from build123d import *

# Parameters (mm, degrees)
SKETCH1_W                      = 12
SKETCH1_H                      = 10.5
BASE_DEPTH                     = 8.25
CONTACT_OPENING_DEPTH          = 9
CONTACT_OPENING_LEAD_IN_SIZE   = 0.5
SKETCH3_W                      = 5.6
SKETCH3_H                      = 3.18
CONTACT_AREA_DEPTH             = 8.5
CONTACT_AREA_LEAD_IN_SIZE      = 0.5
HOLDING_TINES_DEPTH            = 1.75
CONTACT_DEPTH                  = 0.375
CONTACT_PATTERN_COUNT          = 2
CONTACT_PATTERN_PITCH          = 2.5
TH_GROUND_LEGS_DEPTH           = 0.975
TH_GROUND_LEG_SHAPE_DEPTH      = 8.43
TH_GROUND_LEG_SHAPE_DEPTH_BACK = 8.43
TH_TAILS_DEPTH                 = 0.125
TH_TAILS_PATTERN_COUNT         = 2
TH_TAILS_PATTERN_PITCH         = 2


with BuildPart() as part:
    # Sketch1 → Base (new body, symmetric)
    with BuildSketch(Plane.XY):
        Rectangle(SKETCH1_W, SKETCH1_H)
    extrude(amount=BASE_DEPTH, both=True)

    # Sketch2 → Contact Opening (cut)
    with BuildSketch(Plane.XY.offset(8.25)):
        with BuildLine():
            Line((-2.975, 4.33), (-4.225, 3.08))
            Line((-4.225, 3.08), (-4.225, -2.95))
            ThreePointArc((-4.225, -2.95), (-4.078553391, -3.303553391), (-3.725, -3.45))
            Line((-3.725, -3.45), (3.725, -3.45))
            ThreePointArc((3.725, -3.45), (4.078553391, -3.303553391), (4.225, -2.95))
            Line((4.225, -2.95), (4.225, 3.08))
            Line((4.225, 3.08), (2.975, 4.33))
            Line((2.975, 4.33), (-2.975, 4.33))
        make_face()
    extrude(amount=-CONTACT_OPENING_DEPTH, mode=Mode.SUBTRACT)

    # Contact Opening Lead-in
    contact_opening_lead_in_edges = [part.edges().sort_by_distance(p)[0] for p in [
        (0, 4.33, 8.25),
        (-3.6, 3.705, 8.25),
        (-4.225, 0.065, 8.25),
        (-4.078553391, -3.303553391, 8.25),
        (0, -3.45, 8.25),
        (4.078553391, -3.303553391, 8.25),
        (4.225, 0.065, 8.25),
        (3.6, 3.705, 8.25),
    ]]
    chamfer(contact_opening_lead_in_edges, length=CONTACT_OPENING_LEAD_IN_SIZE)

    # Sketch3 → Contact Area (add)
    with BuildSketch(Plane.XY.offset(-0.75)):
        with Locations((0, 0.44)):
            Rectangle(SKETCH3_W, SKETCH3_H)
    extrude(amount=CONTACT_AREA_DEPTH)

    # Contact Area Lead-in
    contact_area_lead_in_edges = [part.edges().sort_by_distance(p)[0] for p in [
        (-2.8, 0.44, 7.75),
        (0, -1.15, 7.75),
        (2.8, 0.44, 7.75),
        (0, 2.03, 7.75),
    ]]
    chamfer(contact_area_lead_in_edges, length=CONTACT_AREA_LEAD_IN_SIZE)

    # Sketch7 → Holding Tines (add, symmetric)
    with BuildSketch(Plane(origin=(0, 0, 0), x_dir=(1, 0, 0), z_dir=(0, 1, 0))):
        with BuildLine():
            Line((-4.225, -7.75), (-3.215243234, -5.051316752))
            ThreePointArc((-3.215243234, -5.051316752), (-3.027350135, -3.881276433), (-3.307189725, -2.729760924))
            Line((-3.307189725, -2.729760924), (-3.695, -1.9))
            Line((-3.695, -1.9), (-3.853538933, -1.974097279))
            Line((-3.853538933, -1.974097279), (-3.465728658, -2.803858203))
            ThreePointArc((-3.465728658, -2.803858203), (-3.202213044, -3.888201975), (-3.379145712, -4.989989942))
            Line((-3.379145712, -4.989989942), (-4.388902478, -7.688673189))
            Line((-4.388902478, -7.688673189), (-4.225, -7.75))
        make_face()
        with BuildLine():
            Line((4.225, -7.75), (4.388902478, -7.688673189))
            Line((4.388902478, -7.688673189), (3.379145712, -4.989989942))
            ThreePointArc((3.379145712, -4.989989942), (3.202213044, -3.888201975), (3.465728658, -2.803858203))
            Line((3.465728658, -2.803858203), (3.853538933, -1.974097279))
            Line((3.853538933, -1.974097279), (3.695, -1.9))
            Line((3.695, -1.9), (3.307189725, -2.729760924))
            ThreePointArc((3.307189725, -2.729760924), (3.027350135, -3.881276433), (3.215243234, -5.051316752))
            Line((3.215243234, -5.051316752), (4.225, -7.75))
        make_face()
    extrude(amount=HOLDING_TINES_DEPTH, both=True)

    # Sketch8 → Contact (add, symmetric)
    with BuildSketch(Plane(origin=(-1.25, 0, 0), x_dir=(0, 0, -1), z_dir=(1, 0, 0))):
        with BuildLine():
            Line((0.75, 2.03), (-2.695251124, 2.678262825))
            ThreePointArc((-2.695251124, 2.678262825), (-3.57053143, 2.712827451), (-4.418484282, 2.493086043))
            Line((-4.418484282, 2.493086043), (-5.75, 1.93))
            Line((-5.75, 1.93), (-5.681838417, 1.768819981))
            Line((-5.681838417, 1.768819981), (-4.350322699, 2.331906024))
            ThreePointArc((-4.350322699, 2.331906024), (-3.551833763, 2.538829183), (-2.727611475, 2.506280827))
            Line((-2.727611475, 2.506280827), (0.717639649, 1.858018002))
            Line((0.717639649, 1.858018002), (0.75, 2.03))
        make_face()
        with BuildLine():
            Line((-5.681838417, -0.888819981), (-5.75, -1.05))
            Line((-5.75, -1.05), (-4.418484282, -1.613086043))
            ThreePointArc((-4.418484282, -1.613086043), (-3.57053143, -1.832827451), (-2.695251124, -1.798262825))
            Line((-2.695251124, -1.798262825), (0.75, -1.15))
            Line((0.75, -1.15), (0.717639649, -0.978018002))
            Line((0.717639649, -0.978018002), (-2.727611475, -1.626280827))
            ThreePointArc((-2.727611475, -1.626280827), (-3.551833763, -1.658829183), (-4.350322699, -1.451906024))
            Line((-4.350322699, -1.451906024), (-5.681838417, -0.888819981))
        make_face()
    contact = extrude(amount=CONTACT_DEPTH, both=True)

    # Contact Pattern: Contact ×2
    with Locations(*[(i * CONTACT_PATTERN_PITCH, 0, 0) for i in range(1, CONTACT_PATTERN_COUNT)]):
        add(contact)

    # Sketch13 → TH Ground Legs (add, symmetric)
    with BuildSketch(Plane.XY.offset(-2.15)):
        with BuildLine():
            Line((6, -5.25), (6, -5.45))
            ThreePointArc((6, -5.45), (6.112536174, -5.84514538), (6.41637299, -6.121709028))
            Line((6.41637299, -6.121709028), (6.736045017, -6.280484954))
            ThreePointArc((6.736045017, -6.280484954), (7.400291967, -7.129098698), (7.157524757, -8.179066973))
            Line((7.157524757, -8.179066973), (6.527167526, -8.97))
            Line((6.527167526, -8.97), (6.23, -8.73316364))
            Line((6.23, -8.73316364), (6.860357231, -7.942230613))
            ThreePointArc((6.860357231, -7.942230613), (7.029323209, -7.211452694), (6.567007332, -6.620817528))
            Line((6.567007332, -6.620817528), (6.247335304, -6.462041602))
            ThreePointArc((6.247335304, -6.462041602), (5.789554503, -6.045352372), (5.62, -5.45))
            Line((5.62, -5.45), (5.62, -5.25))
            Line((5.62, -5.25), (6, -5.25))
        make_face()
        with BuildLine():
            Line((-5.62, -5.25), (-6, -5.25))
            Line((-6, -5.25), (-6, -5.45))
            ThreePointArc((-6, -5.45), (-6.112536174, -5.84514538), (-6.41637299, -6.121709028))
            Line((-6.41637299, -6.121709028), (-6.736045017, -6.280484954))
            ThreePointArc((-6.736045017, -6.280484954), (-7.400291967, -7.129098698), (-7.157524757, -8.179066973))
            Line((-7.157524757, -8.179066973), (-6.527167526, -8.97))
            Line((-6.527167526, -8.97), (-6.23, -8.73316364))
            Line((-6.23, -8.73316364), (-6.860357231, -7.942230613))
            ThreePointArc((-6.860357231, -7.942230613), (-7.029323209, -7.211452694), (-6.567007332, -6.620817528))
            Line((-6.567007332, -6.620817528), (-6.247335304, -6.462041602))
            ThreePointArc((-6.247335304, -6.462041602), (-5.789554503, -6.045352372), (-5.62, -5.45))
            Line((-5.62, -5.45), (-5.62, -5.25))
        make_face()
    extrude(amount=TH_GROUND_LEGS_DEPTH, both=True)

    # Sketch14 → TH Ground Leg Shape (cut, two sides)
    with BuildSketch(Plane(origin=(0, 0, 0), x_dir=(0, 0, -1), z_dir=(1, 0, 0))) as th_ground_leg_shape_sk:
        with BuildLine():
            Line((3.125, -5.25), (3.125, -9))
            Line((3.125, -9), (1.175, -9))
            Line((1.175, -9), (1.175, -5.25))
            Line((1.175, -5.25), (1.655236252, -8.542172253))
            ThreePointArc((1.655236252, -8.542172253), (2.15, -8.97), (2.644763748, -8.542172253))
            Line((2.644763748, -8.542172253), (3.125, -5.25))
        make_face()
    extrude(amount=TH_GROUND_LEG_SHAPE_DEPTH, mode=Mode.SUBTRACT)
    extrude(th_ground_leg_shape_sk.sketch, amount=-TH_GROUND_LEG_SHAPE_DEPTH_BACK, mode=Mode.SUBTRACT)

    # Sketch15 → TH Tails (add, symmetric)
    with BuildSketch(Plane(origin=(0, 0, -7.4), x_dir=(-1, 0, 0), z_dir=(0, 0, -1))):
        Polygon((-1.58, -5.25), (-0.92, -5.25), (-0.92, -8.1), (-1.041207868, -8.4), (-1.458792132, -8.4), (-1.58, -8.1), align=None)
        Polygon((0.92, -8.1), (1.041207868, -8.4), (1.458792132, -8.4), (1.58, -8.1), (1.58, -5.25), (0.92, -5.25), align=None)
    th_tails = extrude(amount=TH_TAILS_DEPTH, both=True)

    # TH Tails Pattern: TH Tails ×2
    with Locations(*[(0, 0, i * TH_TAILS_PATTERN_PITCH) for i in range(1, TH_TAILS_PATTERN_COUNT)]):
        add(th_tails)


solid = part.part
The model under review builds one solid part; all positions refer to its coordinate system, in mm. A direction names the side the tool comes from. Give positions to 0.01 mm unless a question says otherwise; leave off trailing zeros. Order: outer loops, then holes, each group sorted by start corner. A loop starts at its lowest first (then second) coordinate and runs counter-clockwise, first axis right, second up. Notation, with made-up numbers: M 43.25,-28.5 L 75.25,-28.5 A30 cw 75.25,-1.5 Z; hole C 76,88.25 d8. An arc over 180 degrees is marked long. One line per question, with ' | ' between items. Start each with the question number.
1) Mouldability with a two-part tool opening along Y and no side actions: class faces 1 (the face through (-3.591, 3.714, 3.56)), 2 (the face through (0, 0, -8.25)), 3 (the face through (0, 2.03, 3)), 4 (the face through (6.99, -6.78, -2.9)) as pulls with the +Y half, pulls with the -Y half, needs draft (parallel to the pull), parting line crosses it, or undercut.
2) Clearance check with flat-ended pins moving along their axes: P1, Ø5, axis at y = -0.5, z = -4.5, coming from the -X side; P2, Ø0.5, axis at x = 1.5, y = -7, coming from the +Z side (3 decimals); P3, Ø0.7, axis at x = -1.5, y = -6.5, coming from the -Z side (3 decimals); P4, Ø6, axis at x = 1.5, y = -6.5, coming from the -Z side. State where each tip first meets the part, or that it passes through.
3) Consider section A-A, the plane z = 0.75. State how many separate pieces and enclosed holes the cut face has, then the cut area to 3 significant figures.
4) Consider section D-D, the plane x = -2. Give the boundary of the cut face in (y, z), then the cut area to 3 significant figures.
5) Consider section C-C, the plane z = 6.5. Give the boundary of the cut face in (x, y) (3 decimals), then the cut area to 3 significant figures.
6) For faces 5 (the face through (-3.5, -0.02, 2.32)), 6 (the face through (0, 5.25, 0)), 7 (the face through (3.79, 3.87, 8)), list the 3-axis set-ups (+Z, -Z, +X, -X, +Y, -Y) from which the entire face can be reached by the end or side of a thin tool; tool diameter is ignored.
7) Wall thickness on L1, parallel to X at y = 1, z = 6.75 (3 decimals); L2, parallel to X at y = -1.75, z = 0 (3 decimals); L3, parallel to X at y = -0.25, z = 6 (3 decimals): over which ranges is each line inside the solid? List them lowest first. Write a range as from..to.
8) Consider section B-B, the plane y = -2.25. Give the boundary of the cut face in (x, z) (3 decimals).
Found:
1) face 1: undercut | face 2: needs draft | face 3: undercut | face 4: pulls with the -Y half
2) P1: stops at x = -6 | P2: stops at z = -5.275 | P3: stops at z = -7.525 | P4: stops at z = -8.25
3) separate pieces: 6 | enclosed holes: 1 | area: 80.3 mm²
4) outline: M -5.25,-8.25 L 5.25,-8.25 L 5.25,8.25 L 4.83,8.25 L 4.33,7.75 L 4.33,-0.75 L 2.03,-0.75 L 2.03,7.25 L 1.53,7.75 L -0.65,7.75 L -1.15,7.25 L -1.15,-0.75 L -3.45,-0.75 L -3.45,7.75 L -3.95,8.25 L -5.25,8.25 Z | area: 130 mm²
5) outline: M -6,-5.25 L 6,-5.25 L 6,5.25 L -6,5.25 Z; M -3.944,-1.75 L -3.757,-1.75 L -3.757,1.75 L -3.944,1.75 Z; M -2.8,-1.15 L 2.8,-1.15 L 2.8,2.03 L -2.8,2.03 Z; M 3.757,-1.75 L 3.944,-1.75 L 3.944,1.75 L 3.757,1.75 Z; hole M -4.225,-2.95 A0.5 ccw -3.725,-3.45 L 3.725,-3.45 A0.5 ccw 4.225,-2.95 L 4.225,3.08 L 2.975,4.33 L -2.975,4.33 L -4.225,3.08 Z | area: 81.0 mm²
6) face 5: none | face 6: +Z, -Z, +X, -X, +Y | face 7: +Z
7) L1: x = -6..-4.225, -4.038..-3.851, -2.8..2.8, 3.851..4.038, 4.225..6 | L2: x = -6..-4.225, 4.225..6 | L3: x = -6..-4.225, -3.757..-3.57, -2.8..2.8, 3.57..3.757, 4.225..6
8) outline: M -6,-8.25 L 6,-8.25 L 6,8.25 L 4.725,8.25 L 4.225,7.75 L 4.225,-0.75 L -4.225,-0.75 L -4.225,7.75 L -4.725,8.25 L -6,8.25 Z
